from build123d import *

# Parameters (mm, degrees)
SKETCH2_W           = 203.2
SKETCH2_H           = 57.15
BOSS_EXTRUDE1_DEPTH = 6.35
SKETCH3_W           = 12.7
SKETCH3_H           = 6.35
CUT_EXTRUDE1_DEPTH  = 6.35
SKETCH5_W           = 6.35
SKETCH5_H           = 6.35
CUT_EXTRUDE2_DEPTH  = 6.35
LPATTERN1_COUNT     = 15
LPATTERN1_PITCH     = 12.7
SKETCH6_W           = 6.35
SKETCH6_H           = 6.35
CUT_EXTRUDE3_DEPTH  = 6.35
SKETCH7_W           = 6.35
SKETCH7_H           = 6.35
CUT_EXTRUDE4_DEPTH  = 6.35
LPATTERN2_COUNT     = 4
LPATTERN2_PITCH     = 12.7
SKETCH8_W           = 6.35
SKETCH8_H           = 6.35
CUT_EXTRUDE5_DEPTH  = 6.35
SKETCH9_W           = 6.35
SKETCH9_H           = 6.35
CUT_EXTRUDE6_DEPTH  = 6.35
LPATTERN3_COUNT     = 4
LPATTERN3_PITCH     = 12.7
CUT_EXTRUDE7_DEPTH  = 190.5


with BuildPart() as part:
    # Sketch2 → Boss-Extrude1 (new body)
    with BuildSketch(Plane.XY):
        with Locations((101.6, 28.575)):
            Rectangle(SKETCH2_W, SKETCH2_H)
    extrude(amount=BOSS_EXTRUDE1_DEPTH)

    # Sketch3 → Cut-Extrude1 (cut)
    with BuildSketch(Plane.XZ):
        with Locations((6.35, 3.175)):
            Rectangle(SKETCH3_W, SKETCH3_H)
    extrude(amount=-CUT_EXTRUDE1_DEPTH, mode=Mode.SUBTRACT)

    # Sketch5 → Cut-Extrude2 (cut)
    with BuildSketch(Plane.XZ):
        with Locations((22.225, 3.175)):
            Rectangle(SKETCH5_W, SKETCH5_H)
    cut_extrude2 = extrude(amount=-CUT_EXTRUDE2_DEPTH, mode=Mode.SUBTRACT)

    # LPattern1: Cut-Extrude2 ×15
    with Locations(*[(i * LPATTERN1_PITCH, 0, 0) for i in range(1, LPATTERN1_COUNT)]):
        add(cut_extrude2, mode=Mode.SUBTRACT)

    # Sketch6 → Cut-Extrude3 (cut)
    with BuildSketch(Plane(origin=(203.2, 0, 0), x_dir=(0, 0, -1), z_dir=(1, 0, 0))):
        with Locations((-3.175, 9.525)):
            Rectangle(SKETCH6_W, SKETCH6_H)
    extrude(amount=-CUT_EXTRUDE3_DEPTH, mode=Mode.SUBTRACT)

    # Sketch7 → Cut-Extrude4 (cut)
    with BuildSketch(Plane(origin=(203.2, 0, 0), x_dir=(0, 0, -1), z_dir=(1, 0, 0))):
        with Locations((-3.175, 22.225)):
            Rectangle(SKETCH7_W, SKETCH7_H)
    cut_extrude4 = extrude(amount=-CUT_EXTRUDE4_DEPTH, mode=Mode.SUBTRACT)

    # LPattern2: Cut-Extrude4 ×4
    with Locations(*[(0, i * LPATTERN2_PITCH, 0) for i in range(1, LPATTERN2_COUNT)]):
        add(cut_extrude4, mode=Mode.SUBTRACT)

    # Sketch8 → Cut-Extrude5 (cut)
    with BuildSketch(Plane(origin=(203.2, 0, 0), x_dir=(0, 0, -1), z_dir=(1, 0, 0))):
        with Locations((-3.175, 53.975)):
            Rectangle(SKETCH8_W, SKETCH8_H)
    extrude(amount=-CUT_EXTRUDE5_DEPTH, mode=Mode.SUBTRACT)

    # Sketch9 → Cut-Extrude6 (cut)
    with BuildSketch(Plane.ZY):
        with Locations((3.175, 15.875)):
            Rectangle(SKETCH9_W, SKETCH9_H)
    cut_extrude6 = extrude(amount=-CUT_EXTRUDE6_DEPTH, mode=Mode.SUBTRACT)

    # LPattern3: Cut-Extrude6 ×4
    with Locations(*[(0, i * LPATTERN3_PITCH, 0) for i in range(1, LPATTERN3_COUNT)]):
        add(cut_extrude6, mode=Mode.SUBTRACT)

    # Sketch10 → Cut-Extrude7 (cut)
    with BuildSketch(Plane.ZY.offset(-6.35)):
        Polygon((6.35, 57.15), (6.35, 50.8), (0, 57.15), align=None)
    extrude(amount=-CUT_EXTRUDE7_DEPTH, mode=Mode.SUBTRACT)


solid = part.part
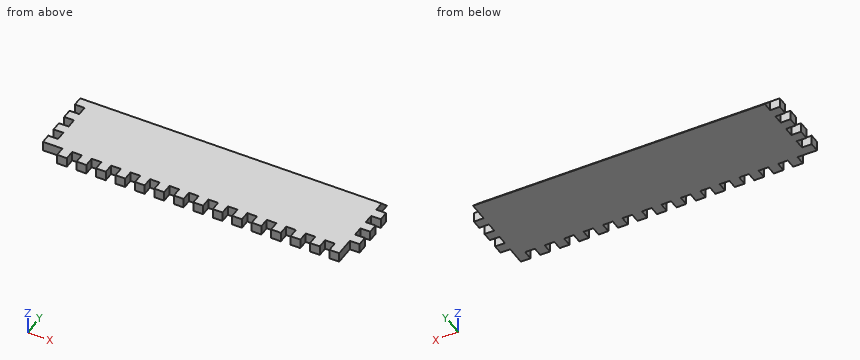
Check sheet for the modelled part. Datum: model origin and axes. Units: mm. Round coordinates to 2 decimals unless told otherwise and drop trailing zeros. Loops run counter-clockwise (first coordinate to the right, second up) from the corner with the lowest first, then second, coordinate; pieces in that order, holes last.
1. Scan lines: probe 1 along X at (y, z) = (43, 2); probe 2 along X at (y, z) = (50.5, 0.5); probe 3 along Y at (x, z) = (107.5, 2). Record each from-to range of solid material in increasing order.
2. Gauge pin test, flat ends, axial feed: pin 1 Ø3 at (y, z) = (22, 1.5) entering from +X; pin 2 Ø1.9 at (x, z) = (161.5, 2.5) entering from -Y; pin 3 Ø2 at (x, z) = (79.5, 4) entering from -Y; pin 4 Ø2 at (y, z) = (17, 5) entering from -X. Record the tip position at first contact, or that the pin passes through.
3. Sectioned sample at C-C on y = 36. Record the boundary of the cut face in (x, z), and give its area (3 significant figures).
4. Sectioned sample at A-A on y = 4. Give the number of separate pieces and of enclosed holes in the cut face, and give its area (3 significant figures).
5. Sectioned sample at B-B on x = 157. Record the boundary of the cut face in (y, z), and give its area (3 significant figures).
Recorded:
1. probe 1: x = 6.35 to 203.2
1. probe 2: x = 0 to 196.85
1. probe 3: y = 0 to 55.15
2. pin 1: stops at x = 196.85
2. pin 2: stops at y = 6.35
2. pin 3: stops at y = 0
2. pin 4: stops at x = 6.35
3. outline: (0, 0) - (196.85, 0) - (196.85, 6.35) - (0, 6.35) - close
3. area: 1,250 mm2
4. separate pieces: 15
4. enclosed holes: 0
4. area: 605 mm2
5. outline: (0, 0) - (57.15, 0) - (50.8, 6.35) - (0, 6.35) - close
5. area: 343 mm2
